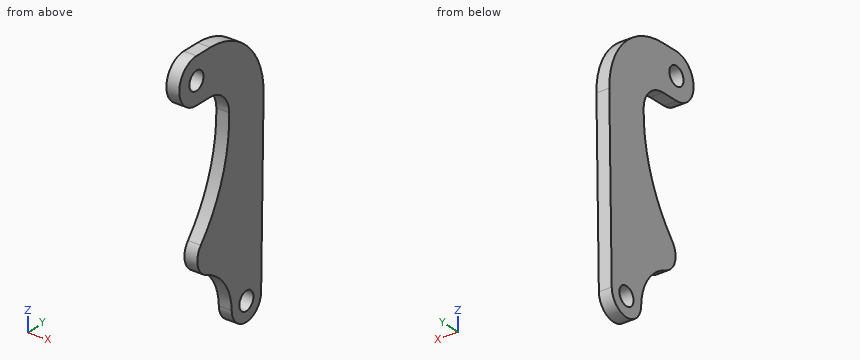
from build123d import *

# Parameters (mm, degrees)
SKETCH1_R           = 2.286
BOSS_EXTRUDE1_DEPTH = 1.5875


with BuildPart() as part:
    # Sketch1 → Boss-Extrude1 (new, symmetric)
    with BuildSketch(Plane(origin=(0, 0, 0), x_dir=(0, 0, -1), z_dir=(1, 0, 0))):
        with BuildLine():
            Line((-5.555690027, 0.078882129), (-5.492947583, 4.497849692))
            ThreePointArc((-5.492947583, 4.497849692), (-0.180708129, 16.793970412), (12.279247772, 21.709656704))
            Line((12.279247772, 21.709656704), (56.556266052, 20.919821075))
            ThreePointArc((56.556266052, 20.919821075), (61.233823705, 16.158078636), (56.556266052, 11.396336198))
            ThreePointArc((56.556266052, 11.396336198), (49.56780942, 9.124706187), (45.041369891, 3.335908885))
            ThreePointArc((45.041369891, 3.335908885), (41.771149469, 0.430257339), (37.509684519, 1.418725347))
            ThreePointArc((37.509684519, 1.418725347), (25.520855431, 8.352797068), (11.854536038, 10.598924348))
            ThreePointArc((11.854536038, 10.598924348), (7.469501812, 8.731884997), (5.61843247, 4.340085435))
            Line((5.61843247, 4.340085435), (5.555690027, -0.078882129))
            ThreePointArc((5.555690027, -0.078882129), (-0.078882129, -5.555690027), (-5.555690027, 0.078882129))
        make_face()
        Circle(SKETCH1_R, mode=Mode.SUBTRACT)
        with Locations((56.471323705, 16.158078636)):
            Circle(SKETCH1_R, mode=Mode.SUBTRACT)
    extrude(amount=BOSS_EXTRUDE1_DEPTH, both=True)


solid = part.part
Model file for the job. Use its own axes, mm. Give positions to 0.01 mm unless a question says otherwise; leave off trailing zeros. Order: outer loops, then holes, each group sorted by start corner. A loop starts at its lowest first (then second) coordinate and runs counter-clockwise, first axis right, second up. Notation, with made-up numbers: M 62.5,16.5 L 96.5,16.5 A16 cw 96.5,25.5 Z; hole C 77.25,53 d11. An arc over 180 degrees is marked long. Put each result on its own line as item: value. Start each with the question number.
(1) Drill centre lines: L1, parallel to Z at x = 0.05, y = 1.5; L2, parallel to Y at x = -0.1, z = 0; L3, parallel to Y at x = -0.25, z = 1.5. Where is each one in solid material? Low to high. Write a range as [from, to].
(2) Band-saw the part on C-C on z = -49. Give the cut face in (x, y).
(3) Band-saw the part on A-A on z = 0. Give the cut face in (x, y).
(4) Pin check, flat tip, straight feed: pin 1 Ø1.5 at (x, y) = (-0.5, 14) entering from +Z. Stop position of the tip, or through.
(5) Band-saw the part on D-D on y = 20.25. Give the cut face in (x, z), then the cut area to 3 significant figures.
(6) Band-saw the part on B-B on x = -1. Count the separate pieces of the cut face and the enclosed holes in it, then the cut area to 3 significant figures.
Results below:
1. L1: z = [-43.78, -37.41], [-5.58, -1.73], [1.73, 5.54]
1. L2: y = [-5.56, -2.29], [2.29, 16.97]
1. L3: y = [-5.35, -1.73], [1.73, 15.37]
2. outline: M -1.59,8.7 L 1.59,8.7 L 1.59,21.05 L -1.59,21.05 Z
3. outline: M -1.59,-5.56 L 1.59,-5.56 L 1.59,-2.29 L -1.59,-2.29 Z; M -1.59,2.29 L 1.59,2.29 L 1.59,16.97 L -1.59,16.97 Z
4. pin 1: stops at z = 3
5. outline: M -1.59,-58.91 L 1.59,-58.91 L 1.59,-4.97 L -1.59,-4.97 Z
5. area: 171 mm2
6. separate pieces: 1
6. enclosed holes: 2
6. area: 945 mm2
